```python
from build123d import *

# Parameters (mm, degrees)
F0_R     = 3
F1_DEPTH = 3


with BuildPart() as f1:
    # F0 (on Front) → F1 (new body)
    with BuildSketch(Plane.XZ):
        with BuildLine():
            Line((-7.750292, 7.75), (-7.749708, -7.75))
            ThreePointArc((-7.749708, -7.75), (0.000292, -15.500292), (7.750292, -7.75))
            Line((7.750292, -7.75), (7.749708, 7.75))
            ThreePointArc((7.749708, 7.75), (-0.000292, 15.499708), (-7.750292, 7.75))
        make_face()
        Circle(F0_R, mode=Mode.SUBTRACT)
    extrude(amount=F1_DEPTH)


solid = f1.part
```
Verification items for the finished model (mm, model axes). Coordinates: 2 decimals unless noted, no trailing zeros. Order: outer loops, then holes, each group sorted by start corner. A loop starts at its lowest first (then second) coordinate and runs counter-clockwise, first axis right, second up. Notation, with made-up numbers: (65, -25) -> (110, -25) arc R25 cw to (110, -5) -> close; hole circle Ø1 at (69.25, -29). An arc over 180 degrees is marked (long way). Answer as CSV lines item,"result". Start each with the question number.
1) Cross-section at A-A, the plane x = 0. Record the boundary of the cut face in (y, z).
2) Gauge pin test, flat ends, axial feed: pin 1 Ø2 at (x, z) = (-1, -5.5) entering from +Y; pin 2 Ø1.5 at (x, y) = (3, -0.5) entering from +Z; pin 3 Ø5 at (x, z) = (0, 0) entering from +Y. Record the tip position at first contact, or that the pin passes through.
3) Cross-section at B-B, the plane z = 0. Record the boundary of the cut face in (x, y), then the cut area to 3 significant figures.
4) Release check for a two-part mould opening along X. For faces 1 (the face through (-3, -1, 0)), 2 (the face through (-0.17, -1.48, -15.5)), 3 (the face through (-0.1, 0, -3.2)) record: released by +X, released by -X, zero draft, split by the parting line, or undercut.
5) Cross-section at C-C, the plane y = -1. Record the boundary of the cut face in (x, z).
6) Cross-section at D-D, the plane x = 5.25. Record the boundary of the cut face in (y, z), then the cut area to 3 significant figures.
7) Material ranges on L1, parallel to Z at x = 0, y = -1.95; L2, parallel to X at y = -0.8, z = 0.5; L3, parallel to X at y = -2.45, z = 2.5, recorded low to high. Write a range as [from, to].
Conclusion:
1,outline,"(-3, -15.5) -> (0, -15.5) -> (0, -3) -> (-3, -3) -> close; (-3, 3) -> (0, 3) -> (0, 15.5) -> (-3, 15.5) -> close"
2,pin 1,"stops at y = 0"
2,pin 2,"stops at z = 15.17"
2,pin 3,"passes through"
3,outline,"(-7.75, -3) -> (-3, -3) -> (-3, 0) -> (-7.75, 0) -> close; (3, -3) -> (7.75, -3) -> (7.75, 0) -> (3, 0) -> close"
3,area,"28.5 mm²"
4,face 1,"undercut"
4,face 2,"split by the parting line"
4,face 3,"zero draft"
5,outline,"(-7.75, -7.75) arc R7.75 ccw to (7.75, -7.75) -> (7.75, 7.75) arc R7.75 ccw to (-7.75, 7.75) -> close; hole circle Ø6 at (0, 0)"
6,outline,"(-3, -13.45) -> (0, -13.45) -> (0, 13.45) -> (-3, 13.45) -> close"
6,area,"80.7 mm²"
7,L1,"z = [-15.5, -3], [3, 15.5]"
7,L2,"x = [-7.75, -2.96], [2.96, 7.75]"
7,L3,"x = [-7.75, -1.66], [1.66, 7.75]"
